```python
from build123d import *

# Parameters (mm, degrees)
F0_W     = 175
F0_H     = 175
F1_DEPTH = 500
F2_R     = 5
F3_R     = 17
F4_W     = 54.523636
F4_H     = 2
F5_DEPTH = 1000


with BuildPart() as f1:
    # F0 (on Front) → F1 (new body, symmetric)
    with BuildSketch(Plane.XZ):
        Polygon((-102.091885, -11.638668), (-102.091885, -99.190576), (97.908115, -99.190576), (97.908115, 100.809424), (-102.091885, 100.809424), (-102.091885, -11.216699), align=None)
        with Locations((-2.091885, 0.809424)):
            Rectangle(F0_W, F0_H, mode=Mode.SUBTRACT)
    extrude(amount=F1_DEPTH, both=True)

    # F2
    f2_edges = [f1.edges().sort_by_distance(p)[0] for p in [
        (-89.591885, 0, -86.690576),
        (-89.591885, 0, 88.309424),
        (85.408115, 0, 88.309424),
        (85.408115, 0, -86.690576),
    ]]
    fillet(f2_edges, radius=F2_R)

    # F3
    f3_edges = [f1.edges().sort_by_distance(p)[0] for p in [
        (97.908115, 0, 100.809424),
        (-102.091885, 0, 100.809424),
        (-102.091885, 0, -99.190576),
        (97.908115, 0, -99.190576),
    ]]
    fillet(f3_edges, radius=F3_R)

    # F4 (on face) → F5 (cut, through all)
    with BuildSketch(Plane.XZ.offset(500)):
        with Locations((70.071755, 99.809424)):
            Rectangle(F4_W, F4_H)
    extrude(amount=-F5_DEPTH, mode=Mode.SUBTRACT)


solid = f1.part
```
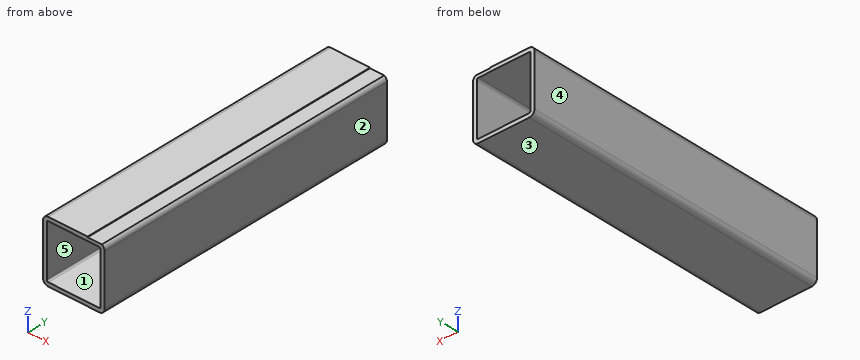
The listing builds one solid part. Answer for the finished solid, in the listing's coordinates (mm). Face numbers are marked on the shaded views. A direction names the side the tool comes from. Coordinates: 2 decimals unless noted, no trailing zeros. Write each loop counter-clockwise with the first axis right and the second up, starting at its lowest first coordinate (ties: lowest second). Pieces come first, ordered by that corner, then holes. Notation, with made-up numbers: M 55.5,-28.75 L 96.5,-28.75 A36 cw 96.5,7.25 Z; hole C 15.25,42 d9. An arc over 180 degrees is marked long. Use a Markdown table: item, result. Add a question column.
1. For a pull along X with two mould halves and no side action, classify the marked faces 1, 2 and 3 as +X half, -X half, draft (parallel to the pull), parting line (faces both ways), or undercut.
2. Straight lines are drawn through the part: line 1 along Z through (x, y) = (37, -23); line 2 along X through (y, z) = (-427, 39); line 3 along Z through (x, y) = (81, 259). For each, find the intervals that lie inside material, in ascending order. Write a range as [from, to].
3. Section C-C (z = 35.5) is taken. Give the vertices of the cut face in (x, y), plus the area to 3 significant figures.
4. Given P1, Ø1, axis at y = -120, z = 99.5, coming from the +X side, flat-ended and moving along its own axis, determine where the tip first touches the part or whether it passes through.
5. Section A-A (x = 57) is taken. Give the vertices of the cut face in (y, z), plus the area to 3 significant figures.
6. Section B-B (y = 202) is taken. Give the vertices of the cut face in (x, z), plus the area to 3 significant figures.
7. Which of the six approach directions +Z, -Z, +X, -X, +Y, -Y give full straight-line access (tool end or side, diameter ignored) to the marked faces 4 and 5?
Data:
| question | item | result |
|---|---|---|
| 1 | face 1 | undercut |
| 1 | face 2 | +X half |
| 1 | face 3 | draft |
| 2 | line 1 | z = [-99.19, -86.69], [88.31, 100.81] |
| 2 | line 2 | x = [-102.09, -89.59], [85.41, 97.91] |
| 2 | line 3 | z = [-99.19, -86.66], [88.27, 98.81] |
| 3 | outline | M -102.09,-500 L -89.59,-500 L -89.59,500 L -102.09,500 Z; M 85.41,-500 L 97.91,-500 L 97.91,500 L 85.41,500 Z |
| 3 | area | 25,000 mm2 |
| 4 | P1 | stops at x = 42.81 |
| 5 | outline | M -500,-99.19 L 500,-99.19 L 500,-86.69 L -500,-86.69 Z; M -500,88.31 L 500,88.31 L 500,98.81 L -500,98.81 Z |
| 5 | area | 23,000 mm2 |
| 6 | outline | M -102.09,-82.19 A17 ccw -85.09,-99.19 L 80.91,-99.19 A17 ccw 97.91,-82.19 L 97.91,83.81 A17 ccw 88.91,98.81 L 42.81,98.81 L 42.81,100.81 L -85.09,100.81 A17 ccw -102.09,83.81 Z; hole M -89.59,-81.69 A5 ccw -84.59,-86.69 L 80.41,-86.69 A5 ccw 85.41,-81.69 L 85.41,83.31 A5 ccw 80.41,88.31 L -84.59,88.31 A5 ccw -89.59,83.31 Z |
| 6 | area | 9,060 mm2 |
| 7 | face 4 | +Z, -Z, -X, +Y, -Y |
| 7 | face 5 | +Y, -Y |
